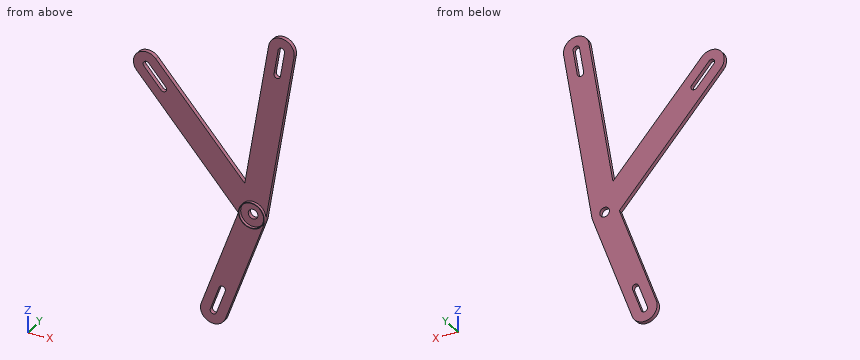
```python
from build123d import *

# Parameters (mm, degrees)
BOSS_EXTRUDE1_DEPTH = 4
BOSS_EXTRUDE2_START = -7
SKETCH3_R           = 12.7
BOSS_EXTRUDE2_DEPTH = 7
SKETCH5_R           = 4.7625
CUT_EXTRUDE1_DEPTH  = 272.846418627
SKETCH6_R           = 12.192
CUT_EXTRUDE2_DEPTH  = 3
SKETCH8_R           = 3.175
CUT_EXTRUDE3_DEPTH  = 272.846418627
CUT_EXTRUDE4_DEPTH  = 272.846418627


with BuildPart() as part:
    # Sketch1 → Boss-Extrude1 (new body)
    with BuildSketch(Plane(origin=(0, 0, 0), x_dir=(1, 0, 0), z_dir=(0, 1, 0))):
        with BuildLine():
            Line((-55.078065391, 65.670374736), (-15.882456002, -41.901827969))
            ThreePointArc((-15.882456002, -41.901827969), (-15.529329867, -43.032283758), (-15.283044075, -44.190718765))
            Line((-15.283044075, -44.190718765), (12.6911511, -214.459876374))
            ThreePointArc((12.6911511, -214.459876374), (2.218090383, -229.050798182), (-12.372831425, -218.577737465))
            Line((-12.372831425, -218.577737465), (-36.044890736, -74.494178583))
            Line((-36.044890736, -74.494178583), (-123.815593368, -172.591431542))
            ThreePointArc((-123.815593368, -172.591431542), (-141.748449811, -173.587754678), (-142.744772948, -155.654898235))
            Line((-142.744772948, -155.654898235), (-42.351793784, -43.450310863))
            Line((-42.351793784, -43.450310863), (-78.943224061, 56.974732054))
            ThreePointArc((-78.943224061, 56.974732054), (-71.358466067, 73.25513273), (-55.078065391, 65.670374736))
        make_face()
    extrude(amount=BOSS_EXTRUDE1_DEPTH)

    # Sketch3 → Boss-Extrude2 (add)
    with BuildSketch(Plane(origin=(0, 4, 0), x_dir=(1, 0, 0), z_dir=(0, 1, 0)).offset(BOSS_EXTRUDE2_START)):
        with Locations(Location((-27.815035337, -46.24964931, 0), (0, 0, 20.02))):
            Circle(SKETCH3_R)
    extrude(amount=BOSS_EXTRUDE2_DEPTH)

    # Sketch5 → Cut-Extrude1 (cut, through all)
    with BuildSketch(Plane(origin=(0, 4, 0), x_dir=(1, 0, 0), z_dir=(0, 1, 0))):
        with Locations(Location((-27.815035337, -46.24964931, 0), (0, 0, 270))):
            Circle(SKETCH5_R)
    extrude(amount=-CUT_EXTRUDE1_DEPTH, mode=Mode.SUBTRACT)

    # Sketch6 → Cut-Extrude2 (cut)
    with BuildSketch(Plane(origin=(0, -3, 0), x_dir=(-1, 0, 0), z_dir=(0, -1, 0))):
        with Locations(Location((27.815035337, -46.24964931, 0), (0, 0, 90))):
            Circle(SKETCH6_R)
    extrude(amount=-CUT_EXTRUDE2_DEPTH, mode=Mode.SUBTRACT)

    # Sketch8 → Cut-Extrude3 (cut, through all)
    with BuildSketch(Plane(origin=(0, 4, 0), x_dir=(1, 0, 0), z_dir=(0, 1, 0))):
        with Locations(Location((-67.010644726, 61.322553395, 0), (0, 0, 270))):
            Circle(SKETCH8_R)
        with Locations(Location((0.159159837, -216.518806919, 0), (0, 0, 270))):
            Circle(SKETCH8_R)
        with Locations(Location((-133.280183158, -164.123164888, 0), (0, 0, 270))):
            Circle(SKETCH8_R)
    extrude(amount=-CUT_EXTRUDE3_DEPTH, mode=Mode.SUBTRACT)

    # Sketch10 → Cut-Extrude4 (cut, through all)
    with BuildSketch(Plane(origin=(0, 4, 0), x_dir=(1, 0, 0), z_dir=(0, 1, 0))):
        with BuildLine():
            Line((-64.027499893, 62.40950873), (-55.331857211, 38.54435006))
            ThreePointArc((-55.331857211, 38.54435006), (-57.228046709, 34.474249891), (-61.298146878, 36.37043939))
            Line((-61.298146878, 36.37043939), (-69.99378956, 60.23559806))
            ThreePointArc((-69.99378956, 60.23559806), (-68.097600062, 64.305698229), (-64.027499893, 62.40950873))
        make_face()
        with BuildLine():
            Line((-135.646330605, -162.006098225), (-118.709797299, -143.076918645))
            ThreePointArc((-118.709797299, -143.076918645), (-114.226583188, -142.827837861), (-113.977502404, -147.311051972))
            Line((-113.977502404, -147.311051972), (-130.91403571, -166.240231552))
            ThreePointArc((-130.91403571, -166.240231552), (-135.397249821, -166.489312336), (-135.646330605, -162.006098225))
        make_face()
        with BuildLine():
            Line((-2.973837978, -217.033539556), (-7.091699069, -191.96955703))
            ThreePointArc((-7.091699069, -191.96955703), (-4.473433889, -188.321826578), (-0.825703437, -190.940091758))
            Line((-0.825703437, -190.940091758), (3.292157653, -216.004074283))
            ThreePointArc((3.292157653, -216.004074283), (0.673892474, -219.651804735), (-2.973837978, -217.033539556))
        make_face()
    extrude(amount=-CUT_EXTRUDE4_DEPTH, mode=Mode.SUBTRACT)


solid = part.part
```
Here's how the part is built. I have some questions about the finished solid (model axes, mm). Coordinates: 2 decimals unless noted, no trailing zeros. Order: outer loops, then holes, each group sorted by start corner. A loop starts at its lowest first (then second) coordinate and runs counter-clockwise, first axis right, second up.
Item 1: If we section it at D-D, the plane x = -19.5: List the corners of the cut face in (y, z) for me, then the cut area to 3 significant figures.
Response values:
outline: (-3, 36.65) - (0, 36.65) - (0, 31.97) - (4, 31.97) - (4, 175.2) - (0, 175.2) - (0, 55.85) - (-3, 55.85) - (-3, 55.17) - (0, 55.17) - (0, 37.33) - (-3, 37.33) - close
area: 577 mm2
Item 2: If we section it at A-A, the plane x = -46: List the corners of the cut face in (y, z) for me, then the cut area to 3 significant figures.
Response values:
outline: (0, -40.76) - (4, -40.76) - (4, 33.44) - (0, 33.44) - close; (0, 47.53) - (4, 47.53) - (4, 85.62) - (0, 85.62) - close
area: 449 mm2
Item 3: I need wall thicknesses on probe 1 along X at (y, z) = (-0.25, 41); probe 2 along X at (y, z) = (3.5, 115.5); probe 3 along Y at (x, z) = (-17, 190). Which ranges of each line are inside material? Lowest first, please.
Response values:
probe 1: x = -39.38 to -38.82, -16.81 to -16.25
probe 2: x = -106.82 to -72.73, -29.31 to -3.57
probe 3: y = 0 to 4
Item 4: If we section it at C-C, the plane y = 2.25: Give the number of separate pieces and of enclosed holes in the cut face, then the cut area to 3 significant figures.
Response values:
separate pieces: 1
enclosed holes: 4
area: 11,000 mm2
Item 5: I'm going to push flat-ended pins straight in: pin 1 Ø7.5 at (x, z) = (-33, 48.5) entering from -Y; pin 2 Ø1 at (x, y) = (-111.5, 3.5) entering from -Z; pin 3 Ø4 at (y, z) = (3, 113) entering from +X. Where does each tip first touch, or does it pass through?
Response values:
pin 1: stops at y = 0
pin 2: stops at z = 120.18
pin 3: stops at x = -3.65
Item 6: If we section it at B-B, the plane z = -50: List the corners of the cut face in (x, y) for me, then the cut area to 3 significant figures.
Response values:
outline: (-76.4, 0) - (-66.26, 0) - (-66.26, 4) - (-76.4, 4) - close; (-59.51, 0) - (-49.37, 0) - (-49.37, 4) - (-59.51, 4) - close
area: 81.1 mm2
